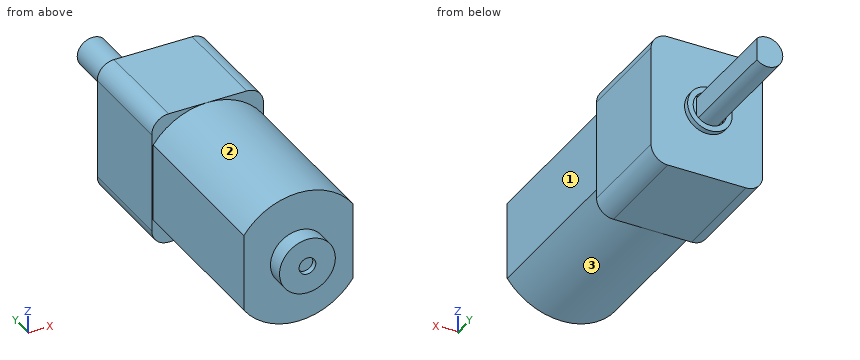
from build123d import *

# Parameters (mm, degrees)
EXTRUDE_1_DEPTH     = 15
SKETCH_2_W          = 10
SKETCH_2_H          = 12
EXTRUDE_2_DEPTH     = 9
FILLET_1_R          = 1.5
SKETCH_3_R          = 2
SKETCH_3_R_2        = 1.5
EXTRUDE_3_DEPTH     = 0.5
EXTRUDE_4_DEPTH     = 10
SKETCH_5_R          = 2.5
EXTRUDE_5_DEPTH     = 1.5
SKETCH_6_R          = 0.75
CUT_EXTRUDE_1_DEPTH = 0.5


with BuildPart() as part:
    # 草图1 → 凸台-拉伸1 (new body)
    with BuildSketch(Plane(origin=(0, 0, 0), x_dir=(1, 0, 0), z_dir=(0, 1, 0))):
        with BuildLine():
            Line((4.873397172, -3.5), (4.873397172, 3.5))
            ThreePointArc((4.873397172, 3.5), (0, 6), (-4.873397172, 3.5))
            Line((-4.873397172, 3.5), (-4.873397172, -3.5))
            ThreePointArc((-4.873397172, -3.5), (0, -6), (4.873397172, -3.5))
        make_face()
    extrude(amount=EXTRUDE_1_DEPTH)

    # 草图2 → 凸台-拉伸2 (add)
    with BuildSketch(Plane(origin=(0, 15, 0), x_dir=(1, 0, 0), z_dir=(0, 1, 0))):
        Rectangle(SKETCH_2_W, SKETCH_2_H)
    extrude(amount=EXTRUDE_2_DEPTH)

    # 圆角1
    fillet_1_edges = [part.edges().sort_by_distance(p)[0] for p in [
        (-5, 19.5, -6),
        (-5, 19.5, 6),
        (5, 19.5, 6),
        (5, 19.5, -6),
    ]]
    fillet(fillet_1_edges, radius=FILLET_1_R)

    # 草图3 → 凸台-拉伸3 (add)
    with BuildSketch(Plane(origin=(0, 24, 0), x_dir=(1, 0, 0), z_dir=(0, 1, 0))):
        with Locations(Location((0, 0, 0), (0, 0, 270))):
            Circle(SKETCH_3_R)
        with Locations(Location((0, 0, 0), (0, 0, 270))):
            Circle(SKETCH_3_R_2, mode=Mode.SUBTRACT)
    extrude(amount=EXTRUDE_3_DEPTH)

    # 草图4 → 凸台-拉伸4 (add)
    with BuildSketch(Plane(origin=(0, 24, 0), x_dir=(1, 0, 0), z_dir=(0, 1, 0))):
        with BuildLine():
            Line((0.943729304, 1), (0.943729304, -1))
            ThreePointArc((0.943729304, -1), (-1.375, 0), (0.943729304, 1))
        make_face()
    extrude(amount=EXTRUDE_4_DEPTH)

    # 草图5 → 凸台-拉伸5 (add)
    with BuildSketch(Plane.XZ):
        with Locations(Location((0, 0, 0), (0, 0, 270))):
            Circle(SKETCH_5_R)
    extrude(amount=EXTRUDE_5_DEPTH)

    # 草图6 → 切除-拉伸1 (cut)
    with BuildSketch(Plane.XZ.offset(1.5)):
        with Locations(Location((0, 0, 0), (0, 0, 270))):
            Circle(SKETCH_6_R)
    extrude(amount=-CUT_EXTRUDE_1_DEPTH, mode=Mode.SUBTRACT)


solid = part.part
Model file for the job. Use its own axes, mm. Face numbers are marked on the shaded views. A direction names the side the tool comes from. Coordinates: 2 decimals unless noted, no trailing zeros. Order: outer loops, then holes, each group sorted by start corner. A loop starts at its lowest first (then second) coordinate and runs counter-clockwise, first axis right, second up. Notation, with made-up numbers: (22.5, 69) -> (33.5, 69) arc R32 cw to (33.5, 106) -> close; hole circle Ø10 at (-6.5, 0.5). An arc over 180 degrees is marked (long way). Return JSON: item names as keys, results as strings. Group by question number.
Item 1: Saw through at C-C on x = -4.5. Write the cut outline in (y, z).
Item 2: Flat gauge pins, fed straight in: P1, Ø2, axis at y = 9, z = 1.5, coming from the -X side; P2, Ø0.6, axis at y = 29.5, z = 0, coming from the +X side; P3, Ø2, axis at x = -1.5, z = 4.5, coming from the +Y side. Where does each tip first touch, or does it go through?
Item 3: Saw through at B-B on y = 6. Write the cut outline in (x, z).
Item 4: Saw through at A-A on z = 0. Write the cut outline in (x, y) (3 decimals), then the cut area to 3 significant figures.
Item 5: Tool access for the marked faces 1, 2 and 3: list every direction of +Z, -Z, +X, -X, +Y, -Y with a clear straight run to the whole face (end or side of a thin tool).
Item 6: Saw through at D-D on y = 25. Write the cut outline in (x, z) (3 decimals), then the cut area to 3 significant figures.
Item 7: Wall check: line 1 along X through (y, z) = (-1.25, 0); line 2 along Y through (x, z) = (3, -3.5); line 3 along Z through (x, y) = (0, 30) (3 decimals). Give the ranges that are in metal, low to high. Write a range as [from, to].
Values found:
{
 "1": {"outline": "(0, -3.97) -> (15, -3.97) -> (15, -5.62) -> (24, -5.62) -> (24, 5.62) -> (15, 5.62) -> (15, 3.97) -> (0, 3.97) -> close"},
 "2": {"P1": "stops at x = -4.87", "P2": "stops at x = 0.94", "P3": "stops at y = 24"},
 "3": {"outline": "(-4.87, -3.5) arc R6 ccw to (4.87, -3.5) -> (4.87, 3.5) arc R6 ccw to (-4.87, 3.5) -> close"},
 "4": {"outline": "(-5, 15) -> (-4.873, 15) -> (-4.873, 0) -> (-2.5, 0) -> (-2.5, -1.5) -> (-0.75, -1.5) -> (-0.75, -1) -> (0.75, -1) -> (0.75, -1.5) -> (2.5, -1.5) -> (2.5, 0) -> (4.873, 0) -> (4.873, 15) -> (5, 15) -> (5, 24) -> (2, 24) -> (2, 24.5) -> (1.5, 24.5) -> (1.5, 24) -> (0.944, 24) -> (0.944, 34) -> (-1.375, 34) -> (-1.375, 24) -> (-1.5, 24) -> (-1.5, 24.5) -> (-2, 24.5) -> (-2, 24) -> (-5, 24) -> close", "area": "267 mm2"},
 "5": {"face 1": "+Z, -Z, +X, -Y", "face 2": "+Z, -Y", "face 3": "-Z, -Y"},
 "6": {"outline": "(0.944, -1) -> (0.944, 1) arc R1.375 ccw (long way) to start", "area": "5.34 mm2"},
 "7": {"line 1": "x = [-2.5, -0.75], [0.75, 2.5]", "line 2": "y = [0, 24]", "line 3": "z = [-1.375, 1.375]"}
}
